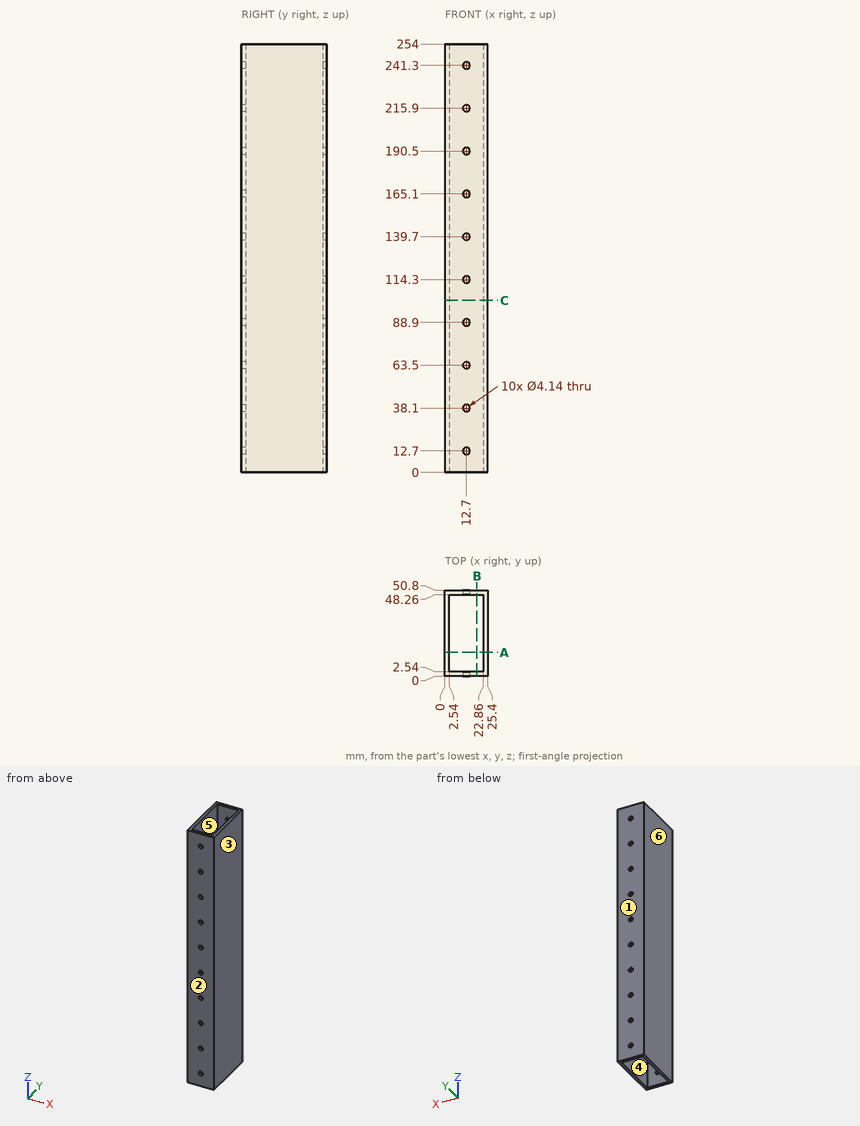
Geometry: see drawing. Coordinates: mm, zero at the bounding-box minimum. A direction names the side the tool comes from. Coordinates: 2 decimals unless noted, no trailing zeros. Loops run counter-clockwise (first coordinate to the right, second up) from the corner with the lowest first, then second, coordinate; pieces in that order, holes last. Notation, with made-up numbers: (59.25, 50) -> (83.25, 50) arc R30 cw to (83.25, 82) -> close; hole circle Ø10 at (18.25, 57.25). An arc over 180 degrees is marked (long way). Write item = value, one per line. Start each with the question number.
Item 1: Mould query, pull axis Y, two halves, no side actions, for the marked faces 1, 2, 3 and 4. Classes: pulls with the +Y half, pulls with the -Y half, needs draft (parallel to the pull), parting line crosses it, or undercut.
Item 2: Cut plane C-C, the plane z = 102. Return loops of the section in (x, y), plus the area to 3 significant figures.
Item 3: Cut plane A-A, the plane y = 14. Return loops of the section in (x, z), plus the area to 3 significant figures.
Item 4: Reachability of the marked faces 5 and 6 from +Z, -Z, +X, -X, +Y, -Y: full face, straight path, thin tool, end or side. Return the list, or none.
Item 5: Material intervals for line 1 (Y direction, x = 3.5, z = 138); line 2 (X direction, y = 39, z = 33); line 3 (X direction, y = 1.9, z = 114.3), sorted ascending.
Item 6: Cut plane B-B, the plane x = 19. Return loops of the section in (y, z), plus the area to 3 significant figures.
Ans:
q1.face_1 = pulls with the +Y half
q1.face_2 = pulls with the -Y half
q1.face_3 = needs draft
q1.face_4 = undercut
q2.outline = (0, 0) -> (25.4, 0) -> (25.4, 50.8) -> (0, 50.8) -> close; hole (2.54, 2.54) -> (22.86, 2.54) -> (22.86, 48.26) -> (2.54, 48.26) -> close
q2.area = 361 mm²
q3.outline = (0, 0) -> (2.54, 0) -> (2.54, 254) -> (0, 254) -> close; (22.86, 0) -> (25.4, 0) -> (25.4, 254) -> (22.86, 254) -> close
q3.area = 1,290 mm²
q4.face_5 = +Z, -Z
q4.face_6 = +Z, -Z, -X, +Y, -Y
q5.line_1 = 0 to 2.54, 48.26 to 50.8
q5.line_2 = 0 to 2.54, 22.86 to 25.4
q5.line_3 = 0 to 10.63, 14.77 to 25.4
q6.outline = (0, 0) -> (2.54, 0) -> (2.54, 254) -> (0, 254) -> close; (48.26, 0) -> (50.8, 0) -> (50.8, 254) -> (48.26, 254) -> close
q6.area = 1,290 mm²
